from build123d import *

# Parameters (mm, degrees)
BOSS_EXTRUDE1_DEPTH = 4.7752
SKETCH4_W           = 4.7752
SKETCH4_H           = 4.7752
CUT_EXTRUDE1_DEPTH  = 5.7752
CUT_EXTRUDE2_DEPTH  = 10


with BuildPart() as part:
    # Sketch1 → Boss-Extrude1 (new body)
    with BuildSketch(Plane.XY):
        with BuildLine():
            Line((-4.5504, 44.7752), (-4.5504, 0.2248))
            ThreePointArc((-4.5504, 0.2248), (-3.085933906, -3.310733906), (0.4496, -4.7752))
            Line((0.4496, -4.7752), (15.4496, -4.7752))
            ThreePointArc((15.4496, -4.7752), (18.985133906, -3.310733906), (20.4496, 0.2248))
            Line((20.4496, 0.2248), (20.4496, 44.7752))
            ThreePointArc((20.4496, 44.7752), (18.985133906, 48.310733906), (15.4496, 49.7752))
            Line((15.4496, 49.7752), (0.4496, 49.7752))
            ThreePointArc((0.4496, 49.7752), (-3.085933906, 48.310733906), (-4.5504, 44.7752))
        make_face()
    extrude(amount=BOSS_EXTRUDE1_DEPTH)

    # Sketch4 → Cut-Extrude1 (cut, through all)
    with BuildSketch(Plane.XY.offset(4.7752)):
        with Locations((-2.1628, 22.5)):
            Rectangle(SKETCH4_W, SKETCH4_H)
    extrude(amount=-CUT_EXTRUDE1_DEPTH, mode=Mode.SUBTRACT)

    # Sketch5 → Cut-Extrude2 (cut)
    with BuildSketch(Plane.XY.offset(4.7752)):
        with BuildLine():
            Line((16.4496, 0.2248), (16.4496, 2.7248))
            ThreePointArc((16.4496, 2.7248), (15.4496, 3.7248), (14.4496, 2.7248))
            Line((14.4496, 2.7248), (14.4496, 0.2248))
            ThreePointArc((14.4496, 0.2248), (15.4496, -0.7752), (16.4496, 0.2248))
        make_face()
    extrude(amount=-CUT_EXTRUDE2_DEPTH, mode=Mode.SUBTRACT)


solid = part.part
Here's how the part is built. I have some questions about the finished solid (model axes, mm). A direction names the side the tool comes from. Round coordinates to 2 decimals unless told otherwise and drop trailing zeros. Loops run counter-clockwise (first coordinate to the right, second up) from the corner with the lowest first, then second, coordinate; pieces in that order, holes last. Notation, with made-up numbers: M 38.5,27.25 L 96.5,27.25 A30 cw 96.5,58.25 Z; hole C -10.5,-32 d10. An arc over 180 degrees is marked long. Write each question's results on one line, items separated by ' | '. Start each with the question number.
(1) Thinking about a two-plate mould opening in X: for faces 1 (the cylindrical face through (18.946, -3.349, 2.354)), 2 (the flat face through (-4.55, 35, 2)), 3 (the cylindrical face through (15.428, -0.775, 2.421)), which applies, pulls with the +X half, pulls with the -X half, needs draft (parallel to the pull), parting line crosses it, or undercut?
(2) I want a section at C-C (x = 19.25). Please give me the cut outline in (y, z).
(3) On a 3-axis mill with a long thin cutter (end or side, diameter ignored), from which of +Z, -Z, +X, -X, +Y, -Y can I reach the whole of each face in a straight line? I mean faces 4 (the cylindrical face through (15.472, 3.725, 2.421)), 5 (the flat face through (8, 23, 4.775)), 6 (the flat face through (-2, 24.888, 2)). Say none if no direction works.
(4) I want a section at A-A (z = 2.9). Please give me the cut outline in (x, y), then the cut area to 3 significant figures.
(5) If I drill on probe 1 along Y at (x, z) = (15.5, 2.85); probe 2 along Y at (x, z) = (-0.25, 3.55); probe 3 along Y at (x, z) = (19.25, 0.95), over which ranges is the centre line in solid material (lowest first)? Write a range as from..to.
(6) Will this pin go through, and if not, where does the flat tip stop? P1, Ø2.5, axis at y = 21.5, z = 1.5, coming from the -X side.
(7) I want a section at B-B (y = 21). Please give me the cut outline in (x, z).
Solved:
1) face 1: pulls with the +X half | face 2: pulls with the -X half | face 3: undercut
2) outline: M -3.02,0 L 48.02,0 L 48.02,4.78 L -3.02,4.78 Z
3) face 4: +Z, -Z | face 5: +Z, +X, -X, +Y, -Y | face 6: +Z, -Z, -X
4) outline: M -4.55,0.22 A5 ccw 0.45,-4.78 L 15.45,-4.78 A5 ccw 20.45,0.22 L 20.45,44.78 A5 ccw 15.45,49.78 L 0.45,49.78 A5 ccw -4.55,44.78 L -4.55,24.89 L 0.22,24.89 L 0.22,20.11 L -4.55,20.11 Z; hole M 14.45,0.22 A1 ccw 16.45,0.22 L 16.45,2.72 A1 ccw 14.45,2.72 Z | area: 1,310 mm²
5) probe 1: y = -4.77..-0.77, 3.72..49.77 | probe 2: y = -4.73..20.11, 24.89..49.73 | probe 3: y = -3.02..48.02
6) P1: stops at x = 0.22
7) outline: M 0.22,0 L 20.45,0 L 20.45,4.78 L 0.22,4.78 Z
